Geometry check sheet. Reference: the model listing, model coordinates, mm. A direction names the side the tool comes from. Coordinates: 2 decimals unless noted, no trailing zeros. Write each loop counter-clockwise with the first axis right and the second up, starting at its lowest first coordinate (ties: lowest second). Pieces come first, ordered by that corner, then holes. Notation, with made-up numbers: (51, -2) -> (56, -2) arc R20 ccw to (56, 21) -> close; hole circle Ø3 at (-11.75, -15.75). An arc over 180 degrees is marked (long way). Answer as CSV lines item,"result".
```python
from build123d import *

# Parameters (mm, degrees)
SKETCH1_W                = 6
SKETCH1_H                = 3
BOSS_EXTRUDE2_DEPTH      = 3
SKETCH4_W                = 2
SKETCH4_H                = 6
BOSS_EXTRUDE3_DEPTH      = 0.75
BOSS_EXTRUDE3_DEPTH_BACK = 0.75


with BuildPart() as part:
    # Sketch1 → Boss-Extrude2 (new body)
    with BuildSketch(Plane(origin=(0, 0, 0), x_dir=(1, 0, 0), z_dir=(0, 1, 0))):
        Polygon((-5, 3.625), (-5, 1), (-3, 1), (-3, -5), (3, -5), (3, 1), (5, 1), (5, 3.625), (3.428571429, 5), (-3.428571429, 5), align=None)
        with Locations((0, -6.5)):
            Rectangle(SKETCH1_W, SKETCH1_H)
        Polygon((-5, 3.625), (-8, 1), (-5, 1), align=None)
        Polygon((0, 8), (-3.428571429, 5), (3.428571429, 5), align=None)
        Polygon((8, 1), (5, 3.625), (5, 1), align=None)
    extrude(amount=BOSS_EXTRUDE2_DEPTH)

    # Sketch4 → Boss-Extrude3 (add, two sides)
    with BuildSketch(Plane(origin=(0, 1.5, 0), x_dir=(1, 0, 0), z_dir=(0, 1, 0))) as boss_extrude3_sk:
        Polygon((10, -5), (10, 5), (5, 5), (5, 3.625), (8, 1), (5, 1), (5, -5), align=None)
        with Locations((4, -2)):
            Rectangle(SKETCH4_W, SKETCH4_H)
        Polygon((3.428571429, 5), (5, 5), (5, 10), (-5, 10), (-5, 5), (-3.428571429, 5), (0, 8), align=None)
        Polygon((-5, 3.625), (-5, 5), (-10, 5), (-10, -5), (-5, -5), (-5, 1), (-8, 1), align=None)
        Polygon((-5, 3.625), (-3.428571429, 5), (-5, 5), align=None)
        Polygon((5, 3.625), (5, 5), (3.428571429, 5), align=None)
        with Locations((-4, -2)):
            Rectangle(SKETCH4_W, SKETCH4_H)
        Polygon((5, -10), (5, -5), (3, -5), (3, -8), (-3, -8), (-3, -5), (-5, -5), (-5, -10), align=None)
    extrude(amount=BOSS_EXTRUDE3_DEPTH)
    extrude(boss_extrude3_sk.sketch, amount=-BOSS_EXTRUDE3_DEPTH_BACK)


solid = part.part
```
Item 1: Cross-section at B-B, the plane y = 2. Record the cut outline in (x, z), plus the area to 3 significant figures.
Responses:
outline,"(-10, -5) -> (-5, -5) -> (-5, -10) -> (5, -10) -> (5, -5) -> (10, -5) -> (10, 5) -> (5, 5) -> (5, 10) -> (-5, 10) -> (-5, 5) -> (-10, 5) -> close"
area,"300 mm2"
Item 2: Cross-section at A-A, the plane z = 6.25. Record the cut outline in (x, y).
Responses:
outline,"(-5, 0.75) -> (-3, 0.75) -> (-3, 0) -> (3, 0) -> (3, 0.75) -> (5, 0.75) -> (5, 2.25) -> (3, 2.25) -> (3, 3) -> (-3, 3) -> (-3, 2.25) -> (-5, 2.25) -> close"
Item 3: Thickness scan on probe 1 along X at (y, z) = (0.5, 3.25); probe 2 along Y at (x, z) = (-6.25, 3.25); probe 3 along Z at (x, y) = (5, 2.45) (3 decimals). Record the ranges inside material, lowest first.
Responses:
probe 1,"x = -3 to 3"
probe 2,"y = 0.75 to 2.25"
probe 3,"z = -3.625 to -1"
Item 4: Cross-section at C-C, the plane z = -8.5. Record the cut outline in (x, y).
Responses:
outline,"(-5, 0.75) -> (5, 0.75) -> (5, 2.25) -> (-5, 2.25) -> close"
Item 5: Depth check by flat-ended pin: pin 1 Ø1.2 at (y, z) = (2, -7) entering from -X; pin 2 Ø1 at (y, z) = (1, -7.5) entering from +X; pin 3 Ø0.6 at (x, y) = (6.5, 2.5) entering from +Z. Enter the tip coordinate at first touch or a pass-through.
Responses:
pin 1,"stops at x = -5"
pin 2,"stops at x = 5"
pin 3,"stops at z = 5"
Item 6: Set-up check for faces 1 (the flat face through (5, 2, 8)), 2 (the flat face through (8, 2, -5)), 3 (the flat face through (-5, 2, -8)): record each of +Z, -Z, +X, -X, +Y, -Y from which the full face is reachable in a straight line by a thin tool's end or side.
Responses:
face 1,"+Z, +X, +Y, -Y"
face 2,"-Z, +X, +Y, -Y"
face 3,"-Z, -X, +Y, -Y"
